Autodesk Fusion 360 part; units mm, degrees
sketch "Skizze1" plane through (0, 0, 0) normal (0, 0, 1) x (1, 0, 0)
  circle A0 centre (0, 0) radius 20
  line L0 (85, 23) -> (-23, 23)
  line L1 (-23, -23) -> (85, -23)
  line L2 (85, -23) -> (85, 23)
  line L3 (85, 23) -> (-23, -6.2235) construction
  line L4 (-23, 6.2235) -> (85, -23) construction
  line L5 (-23, -23) -> (-23, 23)
  line L6 (37.1516, -15.5) -> (68.1516, 15.5) construction
  line L7 (68.1516, -15.5) -> (37.1516, 15.5) construction
  circle A1 centre (37.1516, 15.5) radius 1.65
  circle A2 centre (37.1516, -15.5) radius 1.65
  circle A3 centre (68.1516, -15.5) radius 1.65
  circle A4 centre (68.1516, 15.5) radius 1.65
  circle A5 centre (52.6516, 0) radius 11.5
  line L8 (68.1516, 15.5) -> (66.5016, 15.5)
  line L9 (38.8016, 15.5) -> (37.1516, 15.5)
  line L10 (68.1516, -15.5) -> (68.1516, -13.85)
  line L11 (68.1516, 13.85) -> (68.1516, 15.5)
  line L12 (37.1516, -15.5) -> (38.8016, -15.5)
  line L13 (66.5016, -15.5) -> (68.1516, -15.5)
  line L14 (37.1516, 15.5) -> (37.1516, 13.85)
  line L15 (37.1516, -13.85) -> (37.1516, -15.5)
  line L16 (20, 0) -> (64, 0)
  point P0 (52.6516, 0)
  dimension "d1" = 31
  dimension "d2" = 31
  dimension "d3" = 3.3
  dimension "d4" = 3.3
  dimension "d5" = 3.3
  dimension "d6" = 3.3
  dimension "d7" = 23
extrude "Extrusion1" add sketch "Skizze1" along normal blind 4
sketch "Skizze2" plane through (0, 0, 4) normal (0, 0, 1) x (-1, 0, 0)
  circle A0 centre (-37.1516, 15.5) radius 1.65
  circle A1 centre (0, 0) radius 20
  circle A2 centre (-68.1516, 15.5) radius 1.65
  circle A3 centre (-37.1516, -15.5) radius 1.65
  circle A4 centre (-68.1516, -15.5) radius 1.65
  circle A5 centre (-52.6516, 0) radius 11.5
  line L0 (-85, 23) -> (-85, -23)
  line L1 (-85, -23) -> (23, -23)
  line L2 (23, -23) -> (23, 23)
  line L3 (23, 23) -> (-85, 23)
  line L4 (23, 23) -> (-23, 23)
  line L5 (-23, 23) -> (-23, -23)
  line L6 (-23, -23) -> (23, -23)
  line L7 (23, -23) -> (23, 23)
  line L8 (23, 23) -> (-23, -23) construction
  line L9 (-23, 23) -> (23, -23) construction
extrude "Extrusion2" add sketch "Skizze2" along normal blind 6 contours L1 L2 L3 L4 L5 L6 L7
extrude "Extrusion3" cut 1 faces at (85, -7.6667, 1.3333) along direction (-1, 0, 0) blind 8
fillet "Abrundung1" radius 12.5 4 edges at (-23, 23, 5) (-23, -23, 5) (77, 23, 2) (77, -23, 2)
CAD build for the part. Positions are in the model's coordinates, mm. A direction names the side the tool comes from. Round coordinates to 2 decimals unless told otherwise and drop trailing zeros. Write each loop counter-clockwise with the first axis right and the second up, starting at its lowest first coordinate (ties: lowest second). Pieces come first, ordered by that corner, then holes.
(1) Slice it at A-A, the plane y = -15.5. Write the cut outline in (x, z), and give its area (3 significant figures).
(2) Probe line 1 along X through (y, z) = (0, 1.1); line 2 along X through (y, z) = (-16.5, 0.5); line 3 along X through (y, z) = (16, 1). List the from-to ranges inside material, lowest first.
(3) 3-axis set-ups, long thin cutter, end or side, ignore diameter. For faces 1 (the face through (23, 0, 7)), 2 (the face through (66.94, 14.38, 1.97)): which of +Z, -Z, +X, -X, +Y, -Y reach the whole face in a straight line?
(4) Slice it at B-B, the plane z = 8. Write the cut outline in (x, y).
(5) Slice it at C-C, the plane x = 45. Write the cut outline in (y, z), and give its area (3 significant figures).
(6) Drop flat-ended pins along their axis: P1, Ø4.5, axis at x = 68.15, y = -15.5, coming from the -Z side; P2, Ø4, axis at x = 68.15, y = 15.5, coming from the +Z side; P3, Ø5, axis at y = -9.5, z = 7, coming from the +X side. Give the stop position or say it passes through.
(7) Mould opens along Y. For faces 3 (the face through (67.79, -13.89, 1.97)), 4 (the face through (73.435, 19.241, 2.028)), 5 (the face through (38, 0, 4)) say: pulls with the +Y half, pulls with the -Y half, needs draft (parallel to the pull), parting line crosses it, or undercut.
From the geometry:
1. outline: (-21.96, 0) - (-12.64, 0) - (-12.64, 10) - (-21.96, 10) - close; (12.64, 0) - (35.5, 0) - (35.5, 4) - (23, 4) - (23, 10) - (12.64, 10) - close; (38.8, 0) - (66.5, 0) - (66.5, 4) - (38.8, 4) - close; (69.8, 0) - (75.96, 0) - (75.96, 4) - (69.8, 4) - close
1. area: 382 mm2
2. line 1: x = -23 to -20, 20 to 41.15, 64.15 to 77
2. line 2: x = -21.47 to -11.3, 11.3 to 35.84, 38.46 to 66.84, 69.46 to 75.47
2. line 3: x = -21.72 to -12, 12 to 35.58, 38.72 to 66.58, 69.72 to 75.72
3. face 1: +Z, +X, +Y, -Y
3. face 2: +Z, -Z
4. outline: (-23, -10.5) arc R12.5 ccw to (-10.5, -23) - (23, -23) - (23, 23) - (-10.5, 23) arc R12.5 ccw to (-23, 10.5) - close; hole circle Ø40 at (0, 0)
5. outline: (-23, 0) - (-8.59, 0) - (-8.59, 4) - (-23, 4) - close; (8.59, 0) - (23, 0) - (23, 4) - (8.59, 4) - close
5. area: 115 mm2
6. P1: stops at z = 0
6. P2: stops at z = 4
6. P3: stops at x = 23
7. face 3: undercut
7. face 4: pulls with the +Y half
7. face 5: needs draft
